Geometry: see drawing. Coordinates: mm, zero at the bounding-box minimum. Give positions to 0.01 mm unless a question says otherwise; leave off trailing zeros. Loops run counter-clockwise (first coordinate to the right, second up) from the corner with the lowest first, then second, coordinate; pieces in that order, holes last. Notation, with made-up numbers: M -29.5,15.5 L -17.5,15.5 A21 cw -17.5,24.5 Z; hole C 66.5,-22.75 d6. An arc over 180 degrees is marked long. Use a Markdown table: item, result. Add a question column.
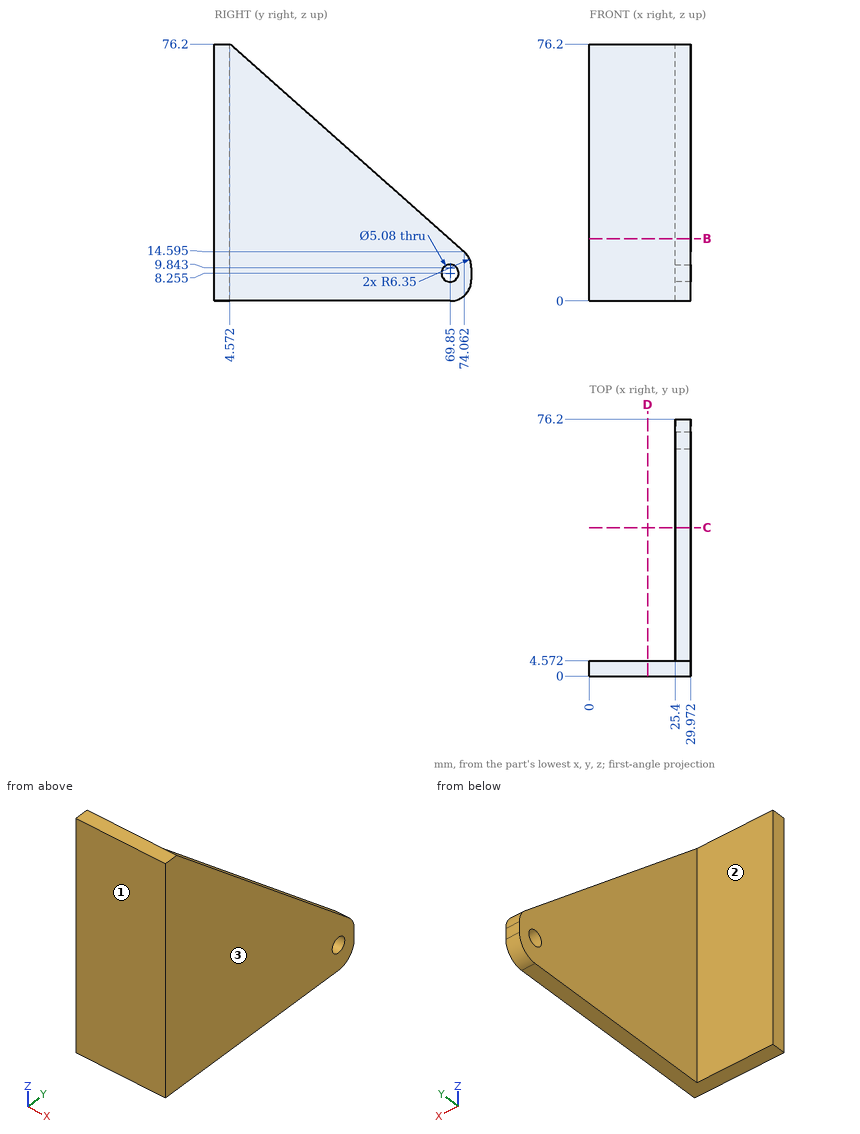
1) Section query D-D, the plane x = 17.25. Return the cut outline in (y, z).
2) Section query C-C, the plane y = 44. Return the cut outline in (x, z).
3) Contact query for flat-ended pins moving along their axis: P1, Ø3, axis at y = 69.85, z = 8.255, coming from the +X side; P2, Ø12, axis at y = 24, z = 61, coming from the -X side; P3, Ø6, axis at x = 15, z = 40, coming from the +Y side. Output: stop coordinate, or through.
4) Section query B-B, the plane z = 18.5. Return the cut outline in (x, y).
5) Ray query, line 1 (Y direction, x = 19.5, z = 56.5); line 2 (X direction, y = 62.5, z = 12); line 3 (Y direction, x = 28.75, z = 27.5) (1 decimal). Return the intervals inside material, ascending. Write a range as [from, to].
6) Pull-direction query (Y, two-part tool) for the marked faces 1, 2 and 3; classes: pulls with the +Y half, pulls with the -Y half, needs draft (parallel to the pull), parting line crosses it, or undercut.
Entries:
| question | item | result |
|---|---|---|
| 1 | outline | M 0,0 L 4.57,0 L 4.57,76.2 L 0,76.2 Z |
| 2 | outline | M 25.4,0 L 29.97,0 L 29.97,41.25 L 25.4,41.25 Z |
| 3 | P1 | passes through |
| 3 | P2 | stops at x = 25.4 |
| 3 | P3 | stops at y = 4.57 |
| 4 | outline | M 0,0 L 29.97,0 L 29.97,69.66 L 25.4,69.66 L 25.4,4.57 L 0,4.57 Z |
| 5 | line 1 | y = [0, 4.57] |
| 5 | line 2 | x = [25.4, 29.97] |
| 5 | line 3 | y = [0, 59.5] |
| 6 | face 1 | pulls with the -Y half |
| 6 | face 2 | pulls with the +Y half |
| 6 | face 3 | needs draft |
